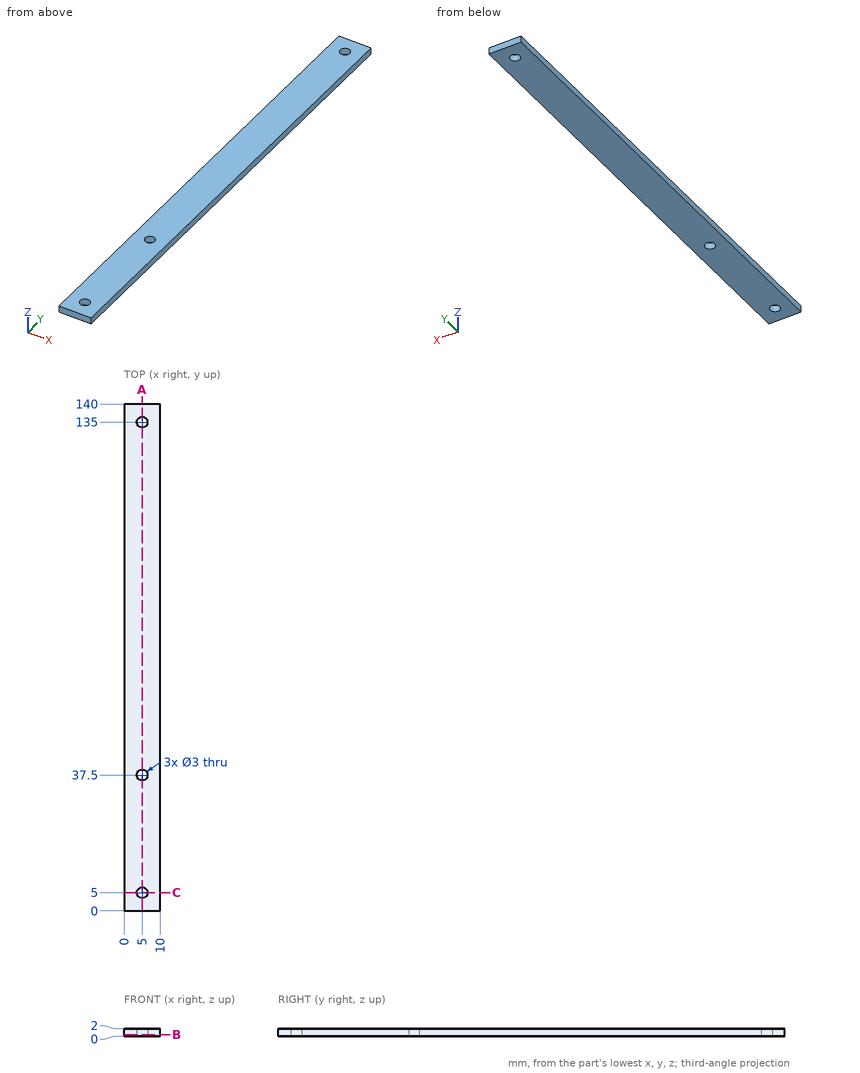
Study the drawing (mm; zero at the part's minimum x, y, z) and answer. Coordinates: 2 decimals unless noted, no trailing zeros. Order: outer loops, then holes, each group sorted by start corner. A loop starts at its lowest first (then second) coordinate and runs counter-clockwise, first axis right, second up. Notation, with made-up numbers: M -30.75,0 L -20.75,0 A30 ccw -20.75,28 Z; hole C -39.5,-37.75 d1. An arc over 180 degrees is marked long. Use CSV: the item, a comma, the result in double quotes.
Q1. Section B-B (z = 0.4) is taken. Determine the outline of the cut face in (x, y), then the cut area to 3 significant figures.
Here are the results:
outline,"M 0,0 L 10,0 L 10,140 L 0,140 Z; hole C 5,5 d3; hole C 5,37.5 d3; hole C 5,135 d3"
area,"1,380 mm2"
Q2. Straight lines are drawn through the part: L1, parallel to Y at x = 5, z = 0.9; L2, parallel to X at y = 37.5, z = 0.55; L3, parallel to Y at x = 6, z = 1.5. For each, find the intervals that lie inside material, in ascending order.
Here are the results:
L1,"0 to 3.5, 6.5 to 36, 39 to 133.5, 136.5 to 140"
L2,"0 to 3.5, 6.5 to 10"
L3,"0 to 3.88, 6.12 to 36.38, 38.62 to 133.88, 136.12 to 140"
Q3. Section A-A (x = 5) is taken. Determine the outline of the cut face in (y, z).
Here are the results:
outline,"M 0,0 L 3.5,0 L 3.5,2 L 0,2 Z; M 6.5,0 L 36,0 L 36,2 L 6.5,2 Z; M 39,0 L 133.5,0 L 133.5,2 L 39,2 Z; M 136.5,0 L 140,0 L 140,2 L 136.5,2 Z"
Q4. Section C-C (y = 5) is taken. Determine the outline of the cut face in (x, z).
Here are the results:
outline,"M 0,0 L 3.5,0 L 3.5,2 L 0,2 Z; M 6.5,0 L 10,0 L 10,2 L 6.5,2 Z"
